Autodesk Inventor part; units mm, degrees
ref_plane "YZ Plane" through (0, 0, 0) normal (1, 0, 0) x (0, 1, 0)
ref_plane "XZ Plane" through (0, 0, 0) normal (0, 1, 0) x (-1, 0, 0)
ref_plane "XY Plane" through (0, 0, 0) normal (0, 0, 1) x (1, 0, 0)
sketch "Sketch1" plane through (0, 0, 0) normal (0, 0, 1) x (1, 0, 0)
  line L0 (37.5, -37.5) -> (-37.5, -37.5)
  line L1 (-37.5, -37.5) -> (-37.5, 37.5)
  line L2 (-37.5, 37.5) -> (37.5, 37.5)
  line L3 (37.5, 37.5) -> (37.5, -37.5)
  line L4 (37.5, -37.5) -> (-37.5, 37.5) construction
  line L5 (-37.5, -37.5) -> (37.5, 37.5) construction
  circle A0 centre (0, 0) radius 7.1
  circle A1 centre (-12, 12.5) radius 2.5
  circle A2 centre (-12, 12.5) radius 1.45
  line L6 (0, 2.5789) -> (0, -2.8298)
  line L7 (-2.79, 0) -> (3.5689, 0)
  circle A3 centre (12, 12.5) radius 2.5
  circle A4 centre (12, 12.5) radius 1.45
  circle A5 centre (-12, -12.5) radius 2.5
  circle A6 centre (-12, -12.5) radius 1.45
  circle A7 centre (12, -12.5) radius 2.5
  circle A8 centre (12, -12.5) radius 1.45
  line L8 (-52.5, 0) -> (52.5, 0)
  dimension "d0" = 75
  dimension "d1" = 75
  dimension "d2" = 14.2
  dimension "d3" = 5
  dimension "d4" = 2.9
  dimension "d7" = 24
  dimension "d10" = 25
extrude "Extrusion1" add sketch "Sketch1" along normal blind 2.5 contours L0 L1 L8 A0 L3 | L8 A0 L1 L2 L3
extrude "Extrusion2" add sketch "Sketch1" along normal blind 6 contours A1 | A3 | A5 | A7
sketch "Sketch2" plane through (37.5, -37.5, 0) normal (1, 0, 0) x (0, 0, -1)
  line L0 (0, -0.0252) -> (0, 75)
  arc A0 (41.0737, 70.0817) -> (39.3854, 64.4916) centre (39.3854, 67.5416) ccw
  arc A1 (39.3854, 10.5916) -> (41.0737, 5.0015) centre (39.3854, 7.5416) ccw
  line L1 (13.8443, 37.5416) -> (29.6757, 37.5416)
  line L2 (0, 75) -> (42, 75)
  line L3 (42, 0) -> (0, 0)
  line L4 (0, 0) -> (0, 75)
  line L5 (39.3854, 64.4916) -> (40.9723, 64.4916)
  line L6 (39.3854, 10.5916) -> (40.9723, 10.5916)
  line L7 (41.0737, 5.0015) -> (41, 5.0015)
  line L8 (41.0737, 70.0817) -> (42, 70.0817)
  line L9 (42, 75) -> (42, 70.0817)
  line L10 (41.9723, 63.4916) -> (41.9723, 11.5916)
  line L11 (42, 4.0015) -> (42, 0)
  arc A2 (41.9723, 63.4916) -> (40.9723, 64.4916) centre (40.9723, 63.4916) ccw
  arc A3 (40.9723, 10.5916) -> (41.9723, 11.5916) centre (40.9723, 11.5916) ccw
  arc A4 (42, 4.0015) -> (41, 5.0015) centre (41, 4.0015) ccw
  point P0 (0, 37.5)
  point P1 (42, 5.0015)
  point P2 (41.07, 4.9991)
  dimension "d18" = 6.1
  dimension "d19" = 6.1
  dimension "d20" = 60
  dimension "d21" = 42
  dimension "d22" = 1
  dimension "d31" = 1
extrude "Extrusion3" add sketch "Sketch2" against normal blind 3 contours L0 L2 L9 L8 A0 L5 A2 L10 A3 L6 A1 A4 L11 L3
sketch "Sketch3" plane through (-37.5, -37.5, 0) normal (-1, 0, 0) x (0, 0, 1)
  line L0 (-42, 4.0015) -> (-42, 0)
  line L1 (-42, 0) -> (0, 0)
  line L2 (0, 75) -> (0, 0)
  line L3 (0, 75) -> (-42, 75)
  line L4 (-42, 75) -> (-42, 70.0817)
  line L5 (-42, 70.0817) -> (-41.0737, 70.0817)
  arc A0 (-39.3854, 64.4916) -> (-41.0737, 70.0817) centre (-39.3854, 67.5416) ccw
  line L6 (-39.3854, 64.4916) -> (-40.9723, 64.4916)
  arc A1 (-40.9723, 64.4916) -> (-41.9723, 63.4916) centre (-40.9723, 63.4916) ccw
  line L7 (-41.9723, 63.4916) -> (-41.9723, 11.5916)
  arc A2 (-41.9723, 11.5916) -> (-40.9723, 10.5916) centre (-40.9723, 11.5916) ccw
  line L8 (-40.9723, 10.5916) -> (-39.3854, 10.5916)
  arc A3 (-41.07, 4.9991) -> (-39.3854, 10.5916) centre (-39.3854, 7.5416) ccw
  arc A4 (-41.07, 4.9991) -> (-42, 4.0015) centre (-41, 4.0015) ccw
  point P0 (0, 37.5)
extrude "Extrusion4" add sketch "Sketch3" against normal blind 3
sketch "Sketch4" plane through (0, 0, 2.5) normal (0, 0, 1) x (1, 0, 0)
  line L0 (15, -15) -> (-15, -15)
  line L1 (-15, -15) -> (-15, 15)
  line L2 (-15, 15) -> (15, 15)
  line L3 (15, 15) -> (15, -15)
  line L4 (15, -15) -> (-15, 15) construction
  line L5 (-15, -15) -> (15, 15) construction
  line L6 (37.5, 37.5) -> (-37.5, 37.5)
  line L7 (-37.5, 37.5) -> (37.5, 37.5)
  line L8 (37.5, 37.5) -> (37.5, -37.5)
  line L9 (37.5, -37.5) -> (-37.5, -37.5)
  line L10 (-37.5, -37.5) -> (-37.5, 37.5)
  point P0 (0, 0)
  dimension "d27" = 30
  dimension "d28" = 30
extrude "Extrusion5" add sketch "Sketch4" along normal up to surface (3.5 mm away)
sketch "Sketch5" plane through (0, 0, 0) normal (0, 0, -1) x (-1, 0, 0)
  line L0 (-34.5, 37.5) -> (-34.5, 32.5817)
  line L1 (34.5, 32.5817) -> (34.5, 37.5)
  line L2 (-34.5, 37.5) -> (34.5, 37.5)
  line L3 (34.5, 37.5) -> (34.5, 35)
  line L4 (34.5, 35) -> (-34.5, 35)
  line L5 (-34.5, 35) -> (-34.5, 37.5)
  point P0 (0, 0)
  dimension "d32" = 2.5
extrude "Extrusion6" add sketch "Sketch5" along normal blind 30
fillet "Fillet2" radius 1 6 edges at (37.5, 37.5, -18) (-37.5, 37.5, -18) (37.5, -37.5, -18) (0, 37.5, -30) (0, 35, -30) (-37.5, -37.5, -18)
properties part number "W(75mm)-camera(FIT0701)"
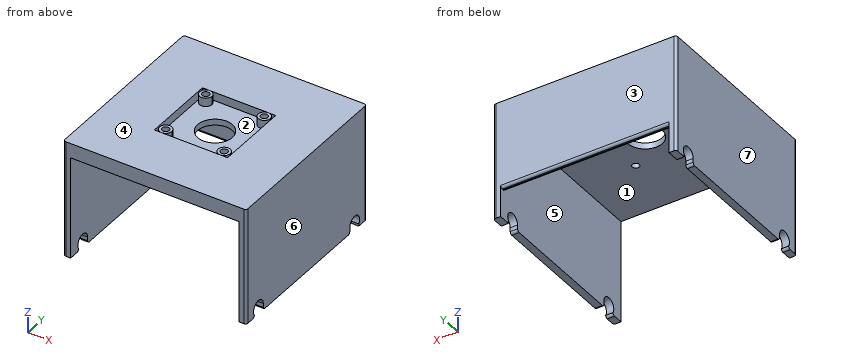
Geometry: final body of the model. Coordinates: model frame, mm. Face numbers are marked on the shaded views. A direction names the side the tool comes from. Give positions to 0.01 mm unless a question says otherwise; leave off trailing zeros. Loops run counter-clockwise (first coordinate to the right, second up) from the corner with the lowest first, then second, coordinate; pieces in that order, holes last. Notation, with made-up numbers: M -31.5,52.25 L -21.5,52.25 A35 cw -21.5,87.25 Z; hole C 73.25,23 d5. An arc over 180 degrees is marked long. Put each result on its own line as item: value.
1) Cut plane D-D, the plane x = 0.5. Return the cut outline in (y, z).
Computed values:
outline: M -37.5,0 L -7.08,0 L -7.08,2.5 L -15,2.5 L -15,6 L -37.5,6 Z; M 7.08,0 L 35,0 L 35,-29 A1 ccw 36,-30 L 36.5,-30 A1 ccw 37.5,-29 L 37.5,6 L 15,6 L 15,2.5 L 7.08,2.5 Z
2) Mould query, pull axis X, two halves, no side actions, for the marked faces 4, 5, 6 and 7. Classes: released by +X, released by -X, zero draft, split by the parting line, or undercut.
Computed values:
face 4: zero draft
face 5: undercut
face 6: released by +X
face 7: released by -X
3) Reachability of the marked faces 1, 2 and 3 from +Z, -Z, +X, -X, +Y, -Y: full face, straight path, thin tool, end or side. Return the list, or none.
Computed values:
face 1: -Z, -Y
face 2: +Z
face 3: +Z, -Z, +X, -X, +Y
4) Material intervals for L1, parallel to X at y = 21.5, z = -6.5; L2, parallel to Y at x = -6.5, z = 4; L3, parallel to Z at x = -12.5, y = -17, sorted ascending. Write a range as from..to.
Computed values:
L1: x = -37.5..-34.5, 34.5..37.5
L2: y = -37.5..-15, 15..37.5
L3: z = 0..6
5) Cut plane B-B, the plane x = -20. Return the cut outline in (y, z).
Computed values:
outline: M -37.5,0 L 35,0 L 35,-29 A1 ccw 36,-30 L 36.5,-30 A1 ccw 37.5,-29 L 37.5,6 L -37.5,6 Z
6) Cut plane C-C, the plane z = -17. Return the cut outline in (x, y).
Computed values:
outline: M -37.5,-36.5 A1 ccw -36.5,-37.5 L -34.5,-37.5 L -34.5,35 L 34.5,35 L 34.5,-37.5 L 36.5,-37.5 A1 ccw 37.5,-36.5 L 37.5,36.5 A1 ccw 36.5,37.5 L -36.5,37.5 A1 ccw -37.5,36.5 Z
7) First-contact query: P1, Ø3.5, axis at x = -36, y = -4.5, coming from the -Z side; P2, Ø8, axis at x = -13.5, y = -17, coming from the -Z side. Flat tips, straight axial feed; report the tip coordinate or a pass-through.
Computed values:
P1: stops at z = -41.97
P2: stops at z = 0
8) Cut plane A-A, the plane y = 0. Return the cut outline in (x, z), plus the area to 3 significant figures.
Computed values:
outline: M -37.5,-41.97 L -34.5,-41.97 L -34.5,0 L -7.1,0 L -7.1,2.5 L -15,2.5 L -15,6 L -37.5,6 Z; M 7.1,0 L 34.5,0 L 34.5,-41.97 L 37.5,-41.97 L 37.5,6 L 15,6 L 15,2.5 L 7.1,2.5 Z
area: 561 mm^2
